Geometry check sheet. Reference: the model listing, model coordinates, mm. A direction names the side the tool comes from. Round coordinates to 2 decimals unless told otherwise and drop trailing zeros. Write each loop counter-clockwise with the first axis right and the second up, starting at its lowest first coordinate (ties: lowest second). Pieces come first, ordered by that corner, then holes.
Item 1: Access from +Z, -Z, +X, -X, +Y, -Y to the whole of each face (thin tool, end or side, straight path). Record for faces 4 (the face through (-296, 197, 0)), 5 (the face through (-591.126, 257.535, 8.874)).
Item 2: Depth check by flat-ended pin: P1, Ø5.5, axis at x = -300.5, z = 10.5, coming from the +Y side; P2, Ø1.5, axis at y = 134.5, z = 16, coming from the -X side. Enter the tip coordinate at first touch or a pass-through.
Item 3: Draft check along X on faces 1 (the face through (0, 339, 9)), 2 (the face through (-437.465, 390.874, 8.874)), 3 (the face through (-600, 199, 9)). Enter one of: pulls with the +X half, pulls with the -X half, needs draft (parallel to the pull), parting line crosses it, or undercut.
Item 4: Scan lines: probe 1 along Y at (x, z) = (-455, 17); probe 2 along X at (y, z) = (273, 7). Record each from-to range of solid material in increasing order.
Item 5: Cross-section at A-A (x = -453). Enter the section's corners in (y, z), then the cut area to 3 significant figures.
from build123d import *

# Parameters (mm, degrees)
F0_W          = 400
F0_H          = 18
F1_DEPTH      = 600
F3_DEPTH      = 18
F3_DEPTH_BACK = 25


with BuildPart() as f1:
    # F0 (on Right) → F1 (new body)
    with BuildSketch(Plane.YZ):
        with Locations((200, 9)):
            Rectangle(F0_W, F0_H)
    extrude(amount=-F1_DEPTH)

    # F2 (on Top) → F3 (cut, two sides)
    with BuildSketch(Plane.XY) as f3_sk:
        Polygon((-300, 400), (-310, 400), (-315, 382), (-300, 382), (-285, 382), (-290, 400), align=None)
        Polygon((-150, 400), (-160, 400), (-165, 382), (-135, 382), (-140, 400), align=None)
        Polygon((-450, 400), (-460, 400), (-465, 382), (-435, 382), (-440, 400), align=None)
        Polygon((-600, 280), (-600, 270), (-600, 260), (-582, 255), (-582, 270), (-582, 285), align=None)
        Polygon((-582, 145), (-600, 140), (-600, 130), (-600, 120), (-582, 115), (-582, 130), align=None)
        Polygon((0, 270), (0, 280), (-18, 285), (-18, 270), (-18, 255), (0, 260), align=None)
        Polygon((-18, 115), (0, 120), (0, 130), (0, 140), (-18, 145), (-18, 130), align=None)
    extrude(amount=F3_DEPTH, mode=Mode.SUBTRACT)
    extrude(f3_sk.sketch, amount=-F3_DEPTH_BACK, mode=Mode.SUBTRACT)


solid = f1.part
Resolved:
1. face 4: -Z, +X, -X, +Y, -Y
1. face 5: +Z, -Z
2. P1: stops at y = 382
2. P2: stops at x = -582
3. face 1: pulls with the +X half
3. face 2: undercut
3. face 3: pulls with the -X half
4. probe 1: y = 0 to 382
4. probe 2: x = -582 to -18
5. outline: (0, 0) - (382, 0) - (382, 18) - (0, 18) - close
5. area: 6,880 mm2
